Check sheet for the modelled part. Datum: model origin and axes. Units: mm. Round coordinates to 2 decimals unless told otherwise and drop trailing zeros. Write each loop counter-clockwise with the first axis right and the second up, starting at its lowest first coordinate (ties: lowest second). Pieces come first, ordered by that corner, then holes. Notation, with made-up numbers: M 77.25,41 L 136.25,41 A12 cw 136.25,58 Z; hole C 72.5,-7.75 d9. An arc over 180 degrees is marked long. One line per item, written item: value.
from build123d import *

# Parameters (mm, degrees)
SKETCH_1_R          = 5
EXTRUDE_1_DEPTH     = 8
SKETCH_2_R          = 2
CUT_EXTRUDE_1_DEPTH = 8


with BuildPart() as part:
    # 草图1 → 凸台-拉伸1 (new body)
    with BuildSketch(Plane.XY):
        with BuildLine():
            Line((-33.201361832, 0), (33.201361832, 0))
            ThreePointArc((33.201361832, 0), (0, 33.201361832), (-33.201361832, 0))
        make_face()
        with Locations((0, 12)):
            Circle(SKETCH_1_R, mode=Mode.SUBTRACT)
    extrude(amount=EXTRUDE_1_DEPTH)

    # 草图2 → 切除-拉伸1 (cut)
    with BuildSketch(Plane.XY.offset(8)):
        with Locations((-28, 10)):
            Circle(SKETCH_2_R)
        with Locations((28, 10)):
            Circle(SKETCH_2_R)
    extrude(amount=-CUT_EXTRUDE_1_DEPTH, mode=Mode.SUBTRACT)


solid = part.part
Q1. Draft check along X on faces 1 (the cylindrical face through (29.908, 10.601, 4.056)), 2 (the cylindrical face through (0.73, 33.193, 3.944)), 3 (the cylindrical face through (-26.092, 10.601, 4.056)), 4 (the flat face through (0, 0, 4)). Enter one of: pulls with the +X half, pulls with the -X half, needs draft (parallel to the pull), parting line crosses it, or undercut.
Completed:
face 1: undercut
face 2: parting line crosses it
face 3: undercut
face 4: needs draft
Q2. Sectioned sample at B-B on z = 6. Enter the section's corners in (x, y), and give its area (3 significant figures).
Completed:
outline: M -33.2,0 L 33.2,0 A33.2 ccw Z; hole C -28,10 d4; hole C 0,12 d10; hole C 28,10 d4
area: 1,630 mm^2
Q3. Sectioned sample at A-A on x = 0. Enter the section's corners in (y, z).
Completed:
outline: M 0,0 L 7,0 L 7,8 L 0,8 Z; M 17,0 L 33.2,0 L 33.2,8 L 17,8 Z
Q4. Depth check by flat-ended pin: P1, Ø3, axis at y = 24, z = 6.5, coming from the -X side. Enter the tip coordinate at first touch or a pass-through.
Completed:
P1: x = -24.41
Q5. Sectioned sample at D-D on x = -28. Enter the section's corners in (y, z).
Completed:
outline: M 0,0 L 8,0 L 8,8 L 0,8 Z; M 12,0 L 17.84,0 L 17.84,8 L 12,8 Z
Q6. Sectioned sample at C-C on y = 10. Enter the section's corners in (x, z), and give its area (3 significant figures).
Completed:
outline: M -31.66,0 L -30,0 L -30,8 L -31.66,8 Z; M -26,0 L -4.58,0 L -4.58,8 L -26,8 Z; M 4.58,0 L 26,0 L 26,8 L 4.58,8 Z; M 30,0 L 31.66,0 L 31.66,8 L 30,8 Z
area: 369 mm^2
Q7. Scan lines: line 1 (Y direction, x = 0, z = 1.5); line 2 (X direction, y = 16, z = 0.75); line 3 (X direction, y = 13, z = 6). Record each from-to range of solid material in increasing order. Write a range as [from, to].
Completed:
line 1: [0, 7], [17, 33.2]
line 2: [-29.09, -3], [3, 29.09]
line 3: [-30.55, -4.9], [4.9, 30.55]
